Verification items for the finished model (mm, model axes). A direction names the side the tool comes from. Give positions to 0.01 mm unless a question says otherwise; leave off trailing zeros. Order: outer loops, then holes, each group sorted by start corner. A loop starts at its lowest first (then second) coordinate and runs counter-clockwise, first axis right, second up.
(1) Scan lines: L1, parallel to X at y = 12, z = 4; L2, parallel to Z at x = -6, y = 1.75; L3, parallel to Y at x = -32, z = 15.8. Record each from-to range of solid material in increasing order.
(2) Access from +Z, -Z, +X, -X, +Y, -Y to the whole of each face (thin tool, end or side, straight path). Record for faces 1 (the face through (5, 7, 12)), 2 (the face through (-18.69, 14.19, -17.26)), 3 (the face through (-1.4, 6.41, 15.23)), 4 (the face through (35.893, 6.595, -0.535)), 5 (the face through (34, 7, 8.5)).
(3) Sectioned sample at C-C on z = 15.5. Count the separate pieces of the cut face and the enclosed holes in it, plus the area to 3 significant figures.
(4) Sectioned sample at A-A on z = 6.5. Record the cut outline in (x, y).
(5) Sectioned sample at B-B on x = -25.5. Record the cut outline in (y, z), plus the area to 3 significant figures.
(6) Gauge pin test, flat ends, axial feed: pin 1 (1.6 mm diameter, centred on x = 34.5, y = 9.5, fed in from +Z); pin 2 (1 mm diameter, centred on x = 4.5, z = 13.5, fed in from +Y); pin 3 (9.5 mm diameter, centred on x = 23.5, y = 5, fed in from -Z); pin 4 (5 mm diameter, centred on x = -18.5, y = 15.5, fed in from -Z). Record the tip position at first contact, or that the pin passes through.
(7) Mould release check, pull along Y, two halves, no side actions. Record for faces 6 (the face through (-28.254, 6.665, -15.514)), 7 (the face through (-33.252, 14.69, -16.687)), 8 (the face through (-7, 18, -16.75)): pulls with the +Y half, pulls with the -Y half, needs draft (parallel to the pull), parting line crosses it, or undercut.
```python
from build123d import *

# Parameters (mm, degrees)
P_IDAT_VYSUNUT_M1_DEPTH  = 13
P_IDAT_VYSUNUT_M2_DEPTH  = 13
SKICA3_W                 = 6
SKICA3_H                 = 12.5
ODEBRAT_VYSUNUT_M1_DEPTH = 44.857724519
SKICA4_W                 = 24
SKICA4_H                 = 16
ODEBRAT_VYSUNUT_M2_DEPTH = 12
SKICA5_R                 = 0.9
ODEBRAT_VYSUNUT_M3_DEPTH = 5
ZAOBLIT1_R               = 6.5
SKICA6_R                 = 3.75
ODEBRAT_VYSUNUT_M4_DEPTH = 5
SKICA7_R                 = 4.75
ODEBRAT_VYSUNUT_M5_DEPTH = 5
SKICA8_W                 = 4
SKICA8_H                 = 11
ODEBRAT_VYSUNUT_M6_DEPTH = 5
SKICA9_R                 = 4
ODEBRAT_VYSUNUT_M7_DEPTH = 10
SKICA10_R                = 6
P_IDAT_VYSUNUT_M3_DEPTH  = 0.5
SKICA11_R                = 4.5
P_IDAT_VYSUNUT_M4_DEPTH  = 3
P_IDAT_VYSUNUT_M5_REACH  = 49.809
P_IDAT_START             = 3
SKICA15_R                = 1.25
P_IDAT_START_2           = 2
P_IDAT_VYSUNUT_M6_DEPTH  = 2


with BuildPart() as part:
    # Skica1 → Přidat vysunutím1 (new body)
    with BuildSketch(Plane(origin=(0, 0, 0), x_dir=(1, 0, 0), z_dir=(0, 1, 0))):
        Polygon((0, -11), (0, 11), (-3.5, 14.5), (-38.5, 14.5), (-38.5, 16.5), (-2.671572875, 16.5), (2, 11.828427125), (2, -11.828427125), (-2.671572875, -16.5), (-38.5, -16.5), (-38.5, -14.5), (-3.5, -14.5), align=None)
    extrude(amount=P_IDAT_VYSUNUT_M1_DEPTH)

    # Skica2 → Přidat vysunutím2 (add)
    with BuildSketch(Plane.XZ):
        Polygon((-0.171572875, 14), (35, 14), (35, 2), (37.5, 2), (37.5, -3), (2, -3), (2, 11.828427125), align=None)
    extrude(amount=-P_IDAT_VYSUNUT_M2_DEPTH)

    # Skica3 → Odebrat vysunutím1 (cut, through all)
    with BuildSketch(Plane(origin=(0, 13, 0), x_dir=(1, 0, 0), z_dir=(0, 1, 0))):
        with Locations((5, -5.75)):
            Rectangle(SKICA3_W, SKICA3_H)
    extrude(amount=-ODEBRAT_VYSUNUT_M1_DEPTH, mode=Mode.SUBTRACT)

    # Skica4 → Odebrat vysunutím2 (cut)
    with BuildSketch(Plane(origin=(0, 13, 0), x_dir=(1, 0, 0), z_dir=(0, 1, 0))):
        with Locations((21.5, -5)):
            Rectangle(SKICA4_W, SKICA4_H)
    extrude(amount=-ODEBRAT_VYSUNUT_M2_DEPTH, mode=Mode.SUBTRACT)

    # Skica5 → Odebrat vysunutím3 (cut)
    with BuildSketch(Plane(origin=(0, 0, -3), x_dir=(-1, 0, 0), z_dir=(0, 0, -1))):
        with Locations((-34.993787626, 6.555058734)):
            Circle(SKICA5_R)
        with Locations((-8.006314188, 6.5550616)):
            Circle(SKICA5_R)
    extrude(amount=-ODEBRAT_VYSUNUT_M3_DEPTH, mode=Mode.SUBTRACT)

    # Zaoblit1
    zaoblit1_edges = [part.edges().sort_by_distance(p)[0] for p in [
        (-38.5, 0, -15.5),
        (-38.5, 13, -15.5),
        (-38.5, 0, 15.5),
        (-38.5, 13, 15.5),
    ]]
    fillet(zaoblit1_edges, radius=ZAOBLIT1_R - 0.0001)  # a hair under: the kernel refuses the full size

    # Skica6 → Odebrat vysunutím4 (cut)
    with BuildSketch(Plane(origin=(0, 0, -16.5), x_dir=(-1, 0, 0), z_dir=(0, 0, -1))):
        with Locations((32, 6.5)):
            Circle(SKICA6_R)
    extrude(amount=-ODEBRAT_VYSUNUT_M4_DEPTH, mode=Mode.SUBTRACT)

    # Skica7 → Odebrat vysunutím5 (cut)
    with BuildSketch(Plane(origin=(0, 0, 14.5), x_dir=(-1, 0, 0), z_dir=(0, 0, -1))):
        with Locations((32, 6.5)):
            Circle(SKICA7_R)
    extrude(amount=-ODEBRAT_VYSUNUT_M5_DEPTH, mode=Mode.SUBTRACT)

    # Skica8 → Odebrat vysunutím6 (cut)
    with BuildSketch(Plane(origin=(35, 0, 0), x_dir=(0, 0, -1), z_dir=(1, 0, 0))):
        with Locations((-10.5, 7.5)):
            Rectangle(SKICA8_W, SKICA8_H)
    extrude(amount=-ODEBRAT_VYSUNUT_M6_DEPTH, mode=Mode.SUBTRACT)

    # Skica9 → Odebrat vysunutím7 (cut)
    with BuildSketch(Plane.XY.offset(14)):
        with Locations((15, 6.554999832)):
            Circle(SKICA9_R)
    extrude(amount=-ODEBRAT_VYSUNUT_M7_DEPTH, mode=Mode.SUBTRACT)

    # Skica10 → Přidat vysunutím3 (add)
    with BuildSketch(Plane.XY.offset(14)):
        with Locations((27.118831388, 6.554999832)):
            Circle(SKICA10_R)
    extrude(amount=P_IDAT_VYSUNUT_M3_DEPTH)

    # Skica11 → Přidat vysunutím4 (add)
    with BuildSketch(Plane.XY.offset(14.5)):
        with Locations((27.118831388, 6.554999832)):
            Circle(SKICA11_R)
    extrude(amount=P_IDAT_VYSUNUT_M4_DEPTH)

    # Táhnout po křivce1: sweep along a path in Skica14
    with BuildLine(Plane(origin=(0, 0, -16.5), x_dir=(-1, 0, 0), z_dir=(0, 0, -1))) as t_hnout_po_k_ivce1_path:
        Line((5, 13), (32, 13))
        ThreePointArc((32, 13), (32.996059893, 12.923228525), (33.968590866, 12.694727597))
    # Skica12 → Táhnout po křivce1 (sweep)
    with BuildSketch(Plane.ZY.offset(5)):
        Polygon((-14.5, 13), (-16.5, 13), (-18, 15.354528366), (-17.5, 15.354528366), (-15.851162616, 14.2), (-15.148837384, 14.2), (-13.5, 15.354528366), (-13, 15.354528366), align=None)
    sweep(path=t_hnout_po_k_ivce1_path.line)

    # Skica15 → Přidat vysunutím5 (add, up to next)
    with BuildSketch(Plane(origin=(0, 14.2, 0), x_dir=(1, 0, 0), z_dir=(0, 1, 0)).offset(P_IDAT_START), mode=Mode.PRIVATE) as p_idat_vysunut_m5_sk1:
        with Locations(Location((-7.5, 15.5, 0), (0, 0, 270))):
            Circle(SKICA15_R)
    p_idat_vysunut_m5_tool1 = extrude(p_idat_vysunut_m5_sk1.sketch, amount=-P_IDAT_VYSUNUT_M5_REACH, mode=Mode.PRIVATE) - part.part
    add(p_idat_vysunut_m5_tool1.solids().sort_by_distance((-7.5, 17.2, -15.5))[0])

    # Skica16 → Přidat vysunutím6 (add)
    with BuildSketch(Plane(origin=(0, 17.2, 0), x_dir=(1, 0, 0), z_dir=(0, 1, 0)).offset(P_IDAT_START_2)):
        with BuildLine():
            Line((-7.5, 16.75), (-5.5, 16.75))
            ThreePointArc((-5.5, 16.75), (-4.25, 15.5), (-5.5, 14.25))
            Line((-5.5, 14.25), (-7.5, 14.25))
            ThreePointArc((-7.5, 14.25), (-8.75, 15.5), (-7.5, 16.75))
        make_face()
    extrude(amount=-P_IDAT_VYSUNUT_M6_DEPTH)


solid = part.part
```
Ans:
1. L1: x = 0 to 2, 8 to 9.5, 33.5 to 35
1. L2: z = -16.5 to -14.5, 14.5 to 16.5
1. L3: y = 0 to 1.75, 11.25 to 13
2. face 1: +Y, -Y
2. face 2: -Z, +X, -Y
2. face 3: +Z, +Y, -Y
2. face 4: -Z
2. face 5: +X, +Y
3. separate pieces: 2
3. enclosed holes: 1
3. area: 453 mm2
4. outline: (0, 0) - (2, 0) - (2, 13) - (0, 13) - close; (8, 0) - (35, 0) - (35, 13) - (33.5, 13) - (33.5, 1) - (9.5, 1) - (9.5, 13) - (8, 13) - close
5. outline: (0, -16.5) - (13, -16.5) - (15.35, -18) - (15.35, -17.5) - (14.2, -15.85) - (14.2, -15.15) - (15.35, -13.5) - (15.35, -13) - (13, -14.5) - (0, -14.5) - close; (0, 14.5) - (13, 14.5) - (13, 16.5) - (0, 16.5) - close
5. area: 57.5 mm2
6. pin 1: stops at z = 14
6. pin 2: stops at y = 13
6. pin 3: stops at z = -3
6. pin 4: stops at z = -18
7. face 6: undercut
7. face 7: pulls with the +Y half
7. face 8: needs draft
